Autodesk Inventor part; units mm, degrees
ref_plane "YZ Plane" through (0, 0, 0) normal (1, 0, 0) x (0, 1, 0)
ref_plane "XZ Plane" through (0, 0, 0) normal (0, 1, 0) x (-1, 0, 0)
ref_plane "XY Plane" through (0, 0, 0) normal (0, 0, 1) x (1, 0, 0)
sketch "Sketch1" plane through (0, 0, 0) normal (0, 0, 1) x (1, 0, 0)
  line L0 (-23.739, 2.1473) -> (-23.739, 129.1473) construction
  line L1 (-17.389, 2.1473) -> (-17.389, 129.1473)
  line L2 (-30.089, 129.1473) -> (-30.089, 2.1473)
  arc A0 (-30.089, 2.1473) -> (-17.389, 2.1473) centre (-23.739, 2.1473) ccw
  arc A1 (-17.389, 129.1473) -> (-30.089, 129.1473) centre (-23.739, 129.1473) ccw
  circle A2 centre (-23.739, 129.1473) radius 3.175
  circle A3 centre (-23.739, 2.1473) radius 3.175
  circle A4 centre (0, 0) radius 3.175 construction
  point P0 (-23.739, 65.6473)
  dimension "d0" = 127
  dimension "d1" = 12.7
  dimension "d2" = 6.35
  dimension "d3" = 6.35
  dimension "d4" = 6.35
extrude "Extrusion1" add sketch "Sketch1" along normal blind 3.175
equation "\"d3\" = d2"
equation "\"d4\" = d2"
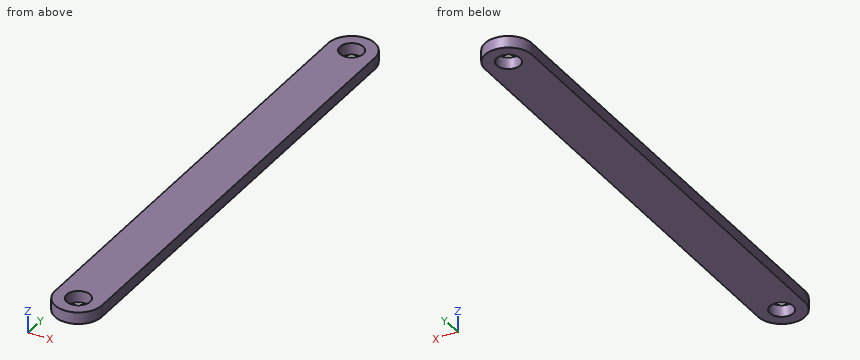
Design review of the part built by this model. Coordinates are the model's own, in mm. Round coordinates to 2 decimals unless told otherwise and drop trailing zeros. Order: outer loops, then holes, each group sorted by start corner. A loop starts at its lowest first (then second) coordinate and runs counter-clockwise, first axis right, second up.
1) Consider section A-A (z = 2.4). State the section outline as (x, y) points (3 decimals).
The answers:
outline: (-30.089, 2.147) arc R6.35 ccw to (-17.389, 2.147) - (-17.389, 129.147) arc R6.35 ccw to (-30.089, 129.147) - close; hole circle Ø6.35 at (-23.739, 2.147); hole circle Ø6.35 at (-23.739, 129.147)
2) For L1, parallel to Y at x = -21.25, z = 0.4; L2, parallel to Y at x = -29.25, z = 1.45; L3, parallel to Y at x = -24.25, z = 1.95, list the stretches that pass through material, from the lowest coordinate up.
The answers:
L1: y = -3.69 to 0.18, 4.12 to 127.18, 131.12 to 134.99
L2: y = -1.01 to 132.3
L3: y = -4.18 to -0.99, 5.28 to 126.01, 132.28 to 135.48
3) Consider section B-B (x = -28.75). State the section outline as (y, z) points (3 decimals).
The answers:
outline: (-1.753, 0) - (133.048, 0) - (133.048, 3.175) - (-1.753, 3.175) - close
4) Clearance check with flat-ended pins moving along their axes: pin 1 Ø2 at (x, y) = (-22, 34.5) entering from -Z; pin 2 Ø1 at (x, z) = (-20.5, 2) entering from +Y. State where each tip first meets the part, or that it passes through.
The answers:
pin 1: stops at z = 0
pin 2: stops at y = 134.88
